Check sheet for the modelled part. Datum: model origin and axes. Units: mm. A direction names the side the tool comes from. Round coordinates to 2 decimals unless told otherwise and drop trailing zeros. Loops run counter-clockwise (first coordinate to the right, second up) from the corner with the lowest first, then second, coordinate; pieces in that order, holes last. Notation, with made-up numbers: (32.25, 21) -> (44.25, 21) arc R18 ccw to (44.25, 34) -> close; hole circle Ø4 at (31, 7.25). An arc over 180 degrees is marked (long way). Return JSON: item names as keys, results as strings.
from build123d import *

# Parameters (mm, degrees)
BOSS_EXTRUDE1_DEPTH = 10
SKETCH2_W           = 1.5
SKETCH2_H           = 2.5
CUT_EXTRUDE1_DEPTH  = 17.9
SKETCH3_R           = 1
CUT_EXTRUDE2_DEPTH  = 37.775671306
CUT_EXTRUDE3_DEPTH  = 1.6
SKETCH5_W           = 2.1
SKETCH5_H           = 3.1
BOSS_EXTRUDE2_DEPTH = 0.3
FILLET1_R           = 0.1
SKETCH6_W           = 4.3
SKETCH6_H           = 3.1
BOSS_EXTRUDE3_DEPTH = 0.2


with BuildPart() as part:
    # Sketch1 → Boss-Extrude1 (new body)
    with BuildSketch(Plane(origin=(0, 0, 0), x_dir=(1, 0, 0), z_dir=(0, 1, 0))):
        Polygon((0, 0), (27.8, 0), (27.8, 12.2), (15.6, 12.2), (15.6, 21.9), (8.6, 21.9), (8.6, 17.25), (0, 17.25), align=None)
    extrude(amount=BOSS_EXTRUDE1_DEPTH)

    # Sketch2 → Cut-Extrude1 (cut)
    with BuildSketch(Plane.XY):
        with Locations((19, 5.05)):
            Rectangle(SKETCH2_W, SKETCH2_H)
        with Locations((21.5, 5.05)):
            Rectangle(SKETCH2_W, SKETCH2_H)
        Polygon((23.25, 6.3), (24, 6.3), (24.6, 5.7), (24.6, 3.8), (23.25, 3.8), align=None)
    extrude(amount=-CUT_EXTRUDE1_DEPTH, mode=Mode.SUBTRACT)

    # Sketch3 → Cut-Extrude2 (cut, through all)
    with BuildSketch(Plane.XY):
        with Locations((22.5, 8.2)):
            Circle(SKETCH3_R)
        with Locations((22.5, 1.8)):
            Circle(SKETCH3_R)
    extrude(amount=-CUT_EXTRUDE2_DEPTH, mode=Mode.SUBTRACT)

    # Sketch4 → Cut-Extrude3 (cut)
    with BuildSketch(Plane(origin=(0, 0, -12.2), x_dir=(-1, 0, 0), z_dir=(0, 0, -1))):
        with BuildLine():
            Line((-24.25, 8.2), (-24.25, 11.165081073))
            Line((-24.25, 11.165081073), (-20.75, 11.165081073))
            Line((-20.75, 11.165081073), (-20.75, 8.2))
            ThreePointArc((-20.75, 8.2), (-22.5, 6.45), (-24.25, 8.2))
        make_face()
        with BuildLine():
            Line((-20.75, -1.165081073), (-20.75, 1.8))
            ThreePointArc((-20.75, 1.8), (-22.5, 3.55), (-24.25, 1.8))
            Line((-24.25, 1.8), (-24.25, -1.165081073))
            Line((-24.25, -1.165081073), (-20.75, -1.165081073))
        make_face()
    extrude(amount=-CUT_EXTRUDE3_DEPTH, mode=Mode.SUBTRACT)

    # Sketch5 → Boss-Extrude2 (add)
    with BuildSketch(Plane.XY):
        Polygon((17.65, 6.9), (17.65, 3.2), (20.35, 3.2), (25.2, 3.2), (25.2, 5.948528137), (24.248528137, 6.9), align=None)
        with Locations((19, 5.05)):
            Rectangle(SKETCH5_W, SKETCH5_H, mode=Mode.SUBTRACT)
        with Locations((21.5, 5.05)):
            Rectangle(SKETCH5_W, SKETCH5_H, mode=Mode.SUBTRACT)
        Polygon((22.95, 6.6), (24.124264069, 6.6), (24.9, 5.824264069), (24.9, 3.5), (22.95, 3.5), align=None, mode=Mode.SUBTRACT)
    extrude(amount=BOSS_EXTRUDE2_DEPTH)

    # Fillet1
    fillet1_edges = [part.edges().sort_by_distance(p)[0] for p in [
        (20.949264069, 6.9, 0.3),
        (17.65, 5.05, 0.3),
        (21.425, 3.2, 0.3),
        (25.2, 4.574264069, 0.3),
        (24.724264069, 6.424264069, 0.3),
        (17.95, 5.05, 0.3),
        (19, 3.5, 0.3),
        (20.05, 5.05, 0.3),
        (19, 6.6, 0.3),
        (20.45, 5.05, 0.3),
        (21.5, 3.5, 0.3),
        (22.55, 5.05, 0.3),
        (21.5, 6.6, 0.3),
        (22.95, 5.05, 0.3),
        (23.925, 3.5, 0.3),
        (24.9, 4.662132034, 0.3),
        (24.512132034, 6.212132034, 0.3),
        (23.537132034, 6.6, 0.3),
    ]]
    fillet(fillet1_edges, radius=FILLET1_R)

    # Sketch6 → Boss-Extrude3 (add)
    with BuildSketch(Plane.XY):
        with Locations((18.45, 8.45)):
            Rectangle(SKETCH6_W, SKETCH6_H)
        with Locations((18.45, 1.55)):
            Rectangle(SKETCH6_W, SKETCH6_H)
    extrude(amount=BOSS_EXTRUDE3_DEPTH)


solid = part.part
Q1. Material ranges on line 1 (Y direction, x = 22.5, z = -3.75); line 2 (X direction, y = 5.5, z = -1.5); line 3 (X direction, y = 7.25, z = -12.75), recorded low to high.
Results list:
{"line 1": "0 to 0.8, 2.8 to 7.2, 9.2 to 10", "line 2": "0 to 18.25, 19.75 to 20.75, 22.25 to 23.25, 24.6 to 27.8", "line 3": "0 to 15.6"}
Q2. Section check A-A (z = -6.25). Record the boundary of the cut face in (x, y), then the cut area to 3 significant figures.
Results list:
{"outline": "(0, 0) -> (27.8, 0) -> (27.8, 10) -> (0, 10) -> close; hole (18.25, 3.8) -> (19.75, 3.8) -> (19.75, 6.3) -> (18.25, 6.3) -> close; hole (20.75, 3.8) -> (22.25, 3.8) -> (22.25, 6.3) -> (20.75, 6.3) -> close; hole circle Ø2 at (22.5, 1.8); hole circle Ø2 at (22.5, 8.2); hole (23.25, 3.8) -> (24.6, 3.8) -> (24.6, 5.7) -> (24, 6.3) -> (23.25, 6.3) -> close", "area": "261 mm^2"}
Q3. Go/stop test with flat-tipped pins: pin 1 (1.3 mm diameter, centred on y = 5.5, z = -6.5, fed in from -X); pin 2 (1 mm diameter, centred on x = 23, y = 2.5, fed in from -Z); pin 3 (1 mm diameter, centred on x = 5.5, y = 7, fed in from +Z); pin 4 (2 mm diameter, centred on x = 20.5, y = 5.5, fed in from -Z). Record where each tip stops, or that it passes through.
Results list:
{"pin 1": "x = 0", "pin 2": "z = -10.6", "pin 3": "z = 0", "pin 4": "z = -12.2"}
Q4. Draft check along X on faces 6 (the flat face through (27.8, 5, -6)), 7 (the flat face through (8.6, 5, -20)), 8 (the cylindrical face through (21.763, 8.876, -5.226)), 9 (the flat face through (20, 5, -12.2)). Enter one of: released by +X, released by -X, zero draft, split by the parting line, or undercut.
Results list:
{"face 6": "released by +X", "face 7": "released by -X", "face 8": "undercut", "face 9": "zero draft"}
Q5. Section check D-D (y = 5). Count the separate pieces of the cut face and the enclosed holes in it, then the cut area to 3 significant figures.
Results list:
{"separate pieces": "4", "enclosed holes": "0", "area": "398 mm^2"}
Q6. Section check C-C (z = -12.75). Record the boundary of the cut face in (x, y).
Results list:
{"outline": "(0, 0) -> (15.6, 0) -> (15.6, 10) -> (0, 10) -> close"}
Q7. Tool access check on faces 1 (the cylindrical face through (22.46, 3.55, -11.41)), 2 (the flat face through (21.7, 9.04, -10.6)), 3 (the flat face through (20.75, 5, -6)), 4 (the flat face through (15.6, 5, -17)), 5 (the flat face through (18, 8, 0.2)). Record the directions out of +Z, -Z, +X, -X, +Y, -Y that give a thin tool (end or side, any length) a straight path to the whole face; none if there is none.
Results list:
{"face 1": "-Z, -Y", "face 2": "-Z, +Y", "face 3": "+Z, -Z", "face 4": "-Z, +X, +Y, -Y", "face 5": "+Z, +X, -X, +Y"}
Q8. Section check B-B (y = 7.5). Record the boundary of the cut face in (x, z), then the cut area to 3 significant figures.
Results list:
{"outline": "(0, -17.25) -> (8.6, -17.25) -> (8.6, -21.9) -> (15.6, -21.9) -> (15.6, -12.2) -> (20.9, -12.2) -> (20.9, -10.6) -> (21.79, -10.6) -> (21.79, 0) -> (20.6, 0) -> (20.6, 0.2) -> (16.3, 0.2) -> (16.3, 0) -> (0, 0) -> close; (23.21, -10.6) -> (24.1, -10.6) -> (24.1, -12.2) -> (27.8, -12.2) -> (27.8, 0) -> (23.21, 0) -> close", "area": "431 mm^2"}
